Geometry: final body of the model. Coordinates: model frame, mm. Give positions to 0.01 mm unless a question says otherwise; leave off trailing zeros. Loops run counter-clockwise (first coordinate to the right, second up) from the corner with the lowest first, then second, coordinate; pieces in that order, holes last. Notation, with made-up numbers: (40.25, 24) -> (68.25, 24) arc R17 ccw to (68.25, 42) -> close; hole circle Ø4 at (38.25, 8.5). An arc over 180 degrees is marked (long way). One line per question, with ' | ' between items. Start each with the question number.
Item 1: Material intervals for line 1 along Z through (x, y) = (-26, 0.9); line 2 along X through (y, z) = (1.6, 88); line 3 along Z through (x, y) = (14, 1), sorted ascending. Write a range as [from, to].
Item 2: Section D-D on z = -68. Return loops of the section in (x, y).
Item 3: Section A-A on x = -85. Return loops of the section in (y, z).
Item 4: Section B-B on y = 0.55. Give the number of separate pieces and of enclosed holes in the cut face, then the cut area to 3 significant figures.
Item 5: Pin query (flat end, axial travel): P1, Ø5.5, axis at x = -14, z = -78, coming from the -Y side; P2, Ø1.5, axis at x = -86, y = 2.5, coming from the -Z side; P3, Ø3.5, axis at x = -103, z = -89, coming from the -Y side (1 decimal); P4, Ø1.5, axis at y = 1, z = 15.5, coming from the +X side. Return the tip coordinate at first contact, or that it passes through.
Item 6: Section C-C on z = 47. Return loops of the section in (x, y).
from build123d import *

# Parameters (mm, degrees)
SKETCH_1_R          = 2.1
EXTRUDE_1_DEPTH     = 3
FILLET_1_R          = 4
SKETCH_2_R          = 2.1
CUT_EXTRUDE_1_DEPTH = 4
EXTRUDE_2_DEPTH     = 3
FILLET_2_R          = 4
SKETCH_5_R          = 1.6
CUT_EXTRUDE_2_DEPTH = 4
FILLET_3_R          = 10
SKETCH_7_R          = 2.1
CUT_EXTRUDE_3_DEPTH = 4
CUT_EXTRUDE_4_DEPTH = 4


with BuildPart() as part:
    # 草图1 → 凸台-拉伸1 (new body)
    with BuildSketch(Plane(origin=(0, 0, 0), x_dir=(1, 0, 0), z_dir=(0, 1, 0))):
        with BuildLine():
            Line((-26, 93), (-96, 93))
            ThreePointArc((-96, 93), (-103.071067812, 95.928932188), (-106, 103))
            Line((-106, 103), (-106, 122.5))
            Line((-106, 122.5), (-130, 122.5))
            Line((-130, 122.5), (-130, -122.5))
            Line((-130, -122.5), (-106, -122.5))
            Line((-106, -122.5), (-106, -103))
            ThreePointArc((-106, -103), (-103.071067812, -95.928932188), (-96, -93))
            Line((-96, -93), (-26, -93))
            Line((-26, -93), (26, -93))
            Line((26, -93), (26, -73))
            Line((26, -73), (-76, -73))
            ThreePointArc((-76, -73), (-97.213203436, -64.213203436), (-106, -43))
            Line((-106, -43), (-106, 43))
            ThreePointArc((-106, 43), (-97.213203436, 64.213203436), (-76, 73))
            Line((-76, 73), (26, 73))
            Line((26, 73), (26, 93))
            Line((26, 93), (-26, 93))
        make_face()
        with Locations((-14, 88)):
            Circle(SKETCH_1_R, mode=Mode.SUBTRACT)
        with Locations((-14, 78)):
            Circle(SKETCH_1_R, mode=Mode.SUBTRACT)
        with Locations((14, 78)):
            Circle(SKETCH_1_R, mode=Mode.SUBTRACT)
        with Locations((14, 88)):
            Circle(SKETCH_1_R, mode=Mode.SUBTRACT)
        with Locations((14, -78)):
            Circle(SKETCH_1_R, mode=Mode.SUBTRACT)
        with Locations((14, -88)):
            Circle(SKETCH_1_R, mode=Mode.SUBTRACT)
        with Locations((-14, -78)):
            Circle(SKETCH_1_R, mode=Mode.SUBTRACT)
        with Locations((-14, -88)):
            Circle(SKETCH_1_R, mode=Mode.SUBTRACT)
    extrude(amount=EXTRUDE_1_DEPTH)

    # 圆角1
    fillet_1_edges = [part.edges().sort_by_distance(p)[0] for p in [
        (26, 1.5, -73),
        (26, 1.5, 73),
        (-130, 1.5, 122.5),
        (-130, 1.5, -122.5),
    ]]
    fillet(fillet_1_edges, radius=FILLET_1_R)

    # 草图2 → 切除-拉伸1 (cut, through all)
    with BuildSketch(Plane(origin=(0, 3, 0), x_dir=(1, 0, 0), z_dir=(0, 1, 0))):
        with Locations((-122, 118.5)):
            Circle(SKETCH_2_R)
        with Locations((-110, 118.5)):
            Circle(SKETCH_2_R)
        with Locations((-122, -118.5)):
            Circle(SKETCH_2_R)
        with Locations((-110, -118.5)):
            Circle(SKETCH_2_R)
    extrude(amount=-CUT_EXTRUDE_1_DEPTH, mode=Mode.SUBTRACT)

    # 草图4 → 凸台-拉伸2 (add)
    with BuildSketch(Plane(origin=(0, 3, 0), x_dir=(1, 0, 0), z_dir=(0, 1, 0))):
        Polygon((-106, 122.5), (16, 93), (-106, 93), align=None)
        Polygon((16, -93), (-106, -93), (-106, -122.5), align=None)
    extrude(amount=-EXTRUDE_2_DEPTH)

    # 圆角2
    fillet_2_edges = [part.edges().sort_by_distance(p)[0] for p in [
        (26, 1.5, 93),
        (-106, 1.5, 122.5),
        (-106, 1.5, -122.5),
        (26, 1.5, -93),
    ]]
    fillet(fillet_2_edges, radius=FILLET_2_R)

    # 草图5 → 切除-拉伸2 (cut, through all)
    with BuildSketch(Plane.XZ):
        with Locations((-110, -15)):
            Circle(SKETCH_5_R)
        with Locations((-110, -5)):
            Circle(SKETCH_5_R)
        with Locations((-110, 5)):
            Circle(SKETCH_5_R)
        with Locations((-110, 15)):
            Circle(SKETCH_5_R)
        with Locations((-26, -77)):
            Circle(SKETCH_5_R)
        with Locations((-36, -77)):
            Circle(SKETCH_5_R)
        with Locations((-46, -77)):
            Circle(SKETCH_5_R)
        with Locations((-56, -77)):
            Circle(SKETCH_5_R)
        with Locations((-56, 77)):
            Circle(SKETCH_5_R)
        with Locations((-46, 77)):
            Circle(SKETCH_5_R)
        with Locations((-36, 77)):
            Circle(SKETCH_5_R)
        with Locations((-26, 77)):
            Circle(SKETCH_5_R)
    extrude(amount=-CUT_EXTRUDE_2_DEPTH, mode=Mode.SUBTRACT)

    # 圆角3
    fillet_3_edges = [part.edges().sort_by_distance(p)[0] for p in [
        (16, 1.5, -93),
        (16, 1.5, 93),
    ]]
    fillet(fillet_3_edges, radius=FILLET_3_R)

    # 草图7 → 切除-拉伸3 (cut, through all)
    with BuildSketch(Plane(origin=(0, 3, 0), x_dir=(1, 0, 0), z_dir=(0, 1, 0))):
        with Locations((-123, -74)):
            Circle(SKETCH_7_R)
        with Locations((-103, -74)):
            Circle(SKETCH_7_R)
        with Locations((-103, -89)):
            Circle(SKETCH_7_R)
        with Locations((-123, -89)):
            Circle(SKETCH_7_R)
        with Locations((-123, 89)):
            Circle(SKETCH_7_R)
        with Locations((-103, 89)):
            Circle(SKETCH_7_R)
        with Locations((-103, 74)):
            Circle(SKETCH_7_R)
        with Locations((-123, 74)):
            Circle(SKETCH_7_R)
    extrude(amount=-CUT_EXTRUDE_3_DEPTH, mode=Mode.SUBTRACT)

    # 草图8 → 切除-拉伸4 (cut, through all)
    with BuildSketch(Plane(origin=(0, 3, 0), x_dir=(1, 0, 0), z_dir=(0, 1, 0))):
        with BuildLine():
            Line((-99.173057144, 103.191305263), (-95.290856101, 86.83060087))
            ThreePointArc((-95.290856101, 86.83060087), (-93.457663057, 84.008976045), (-90.251444241, 82.988033197))
            Line((-90.251444241, 82.988033197), (-38.266720564, 84.80337975))
            ThreePointArc((-38.266720564, 84.80337975), (-33.471381612, 89.251949162), (-37.181429777, 94.639025187))
            Line((-37.181429777, 94.639025187), (-93.048354496, 109.184383027))
            ThreePointArc((-93.048354496, 109.184383027), (-97.805066963, 107.919418235), (-99.173057144, 103.191305263))
        make_face()
        with BuildLine():
            Line((-109, 86.75), (-117, 86.75))
            ThreePointArc((-117, 86.75), (-119.121320344, 85.871320344), (-120, 83.75))
            Line((-120, 83.75), (-120, 79.25))
            ThreePointArc((-120, 79.25), (-119.121320344, 77.128679656), (-117, 76.25))
            Line((-117, 76.25), (-109, 76.25))
            ThreePointArc((-109, 76.25), (-106.878679656, 77.128679656), (-106, 79.25))
            Line((-106, 79.25), (-106, 83.75))
            ThreePointArc((-106, 83.75), (-106.878679656, 85.871320344), (-109, 86.75))
        make_face()
        with BuildLine():
            Line((-109, -76.25), (-117, -76.25))
            ThreePointArc((-117, -76.25), (-119.121320344, -77.128679656), (-120, -79.25))
            Line((-120, -79.25), (-120, -83.75))
            ThreePointArc((-120, -83.75), (-119.121320344, -85.871320344), (-117, -86.75))
            Line((-117, -86.75), (-109, -86.75))
            ThreePointArc((-109, -86.75), (-106.878679656, -85.871320344), (-106, -83.75))
            Line((-106, -83.75), (-106, -79.25))
            ThreePointArc((-106, -79.25), (-106.878679656, -77.128679656), (-109, -76.25))
        make_face()
        with BuildLine():
            Line((-115.138114684, 115), (-115.716605496, 115))
            ThreePointArc((-115.716605496, 115), (-117.80168228, 114.156954985), (-118.714883338, 112.101636537))
            Line((-118.714883338, 112.101636537), (-119.274205372, 95.601636537))
            ThreePointArc((-119.274205372, 95.601636537), (-118.432882515, 93.414923216), (-116.27592753, 92.5))
            Line((-116.27592753, 92.5), (-111.222860446, 92.5))
            ThreePointArc((-111.222860446, 92.5), (-108.869363513, 93.639609669), (-108.30391182, 96.192631877))
            Line((-108.30391182, 96.192631877), (-112.219166057, 112.692631877))
            ThreePointArc((-112.219166057, 112.692631877), (-113.277724353, 114.353496934), (-115.138114684, 115))
        make_face()
        with BuildLine():
            Line((-37.181429777, -94.639025187), (-93.048354496, -109.184383027))
            ThreePointArc((-93.048354496, -109.184383027), (-97.805066963, -107.919418235), (-99.173057144, -103.191305263))
            Line((-99.173057144, -103.191305263), (-95.290856101, -86.83060087))
            ThreePointArc((-95.290856101, -86.83060087), (-93.457663057, -84.008976045), (-90.251444241, -82.988033197))
            Line((-90.251444241, -82.988033197), (-38.266720564, -84.80337975))
            ThreePointArc((-38.266720564, -84.80337975), (-33.471381612, -89.251949162), (-37.181429777, -94.639025187))
        make_face()
        with BuildLine():
            Line((-112.219166057, -112.692631877), (-108.30391182, -96.192631877))
            ThreePointArc((-108.30391182, -96.192631877), (-108.869363513, -93.639609669), (-111.222860446, -92.5))
            Line((-111.222860446, -92.5), (-116.27592753, -92.5))
            ThreePointArc((-116.27592753, -92.5), (-118.432882515, -93.414923216), (-119.274205372, -95.601636537))
            Line((-119.274205372, -95.601636537), (-118.714883338, -112.101636537))
            ThreePointArc((-118.714883338, -112.101636537), (-117.80168228, -114.156954985), (-115.716605496, -115))
            Line((-115.716605496, -115), (-115.138114684, -115))
            ThreePointArc((-115.138114684, -115), (-113.277724353, -114.353496934), (-112.219166057, -112.692631877))
        make_face()
    extrude(amount=-CUT_EXTRUDE_4_DEPTH, mode=Mode.SUBTRACT)


solid = part.part
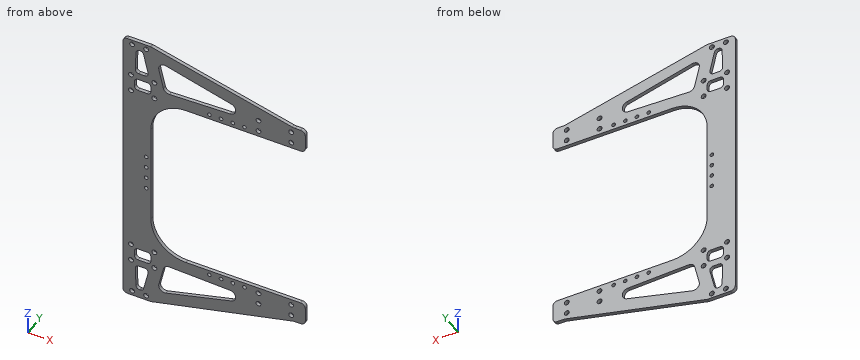
Result sheet:
1) line 1: z = [-103.16, -78.6], [-75.4, -73], [73, 75.4], [78.6, 103.16] | line 2: x = [-130, -124.85], [-121.15, -104.85], [-101.15, -95.57], [-33.78, -16.1], [-11.9, 11.9], [16.1, 26] | line 3: z = [-93.48, -90.1], [-85.9, -80.1], [-75.9, -73], [73, 75.9], [80.1, 85.9], [90.1, 93.48]
2) outline: (-130, 0) -> (-92.58, 0) -> (-92.58, 3) -> (-130, 3) -> close
3) outline: (0, -117.42) -> (3, -117.42) -> (3, -107.09) -> (0, -107.09) -> close; (0, -83.17) -> (3, -83.17) -> (3, -71.62) -> (0, -71.62) -> close; (0, 71.62) -> (3, 71.62) -> (3, 83.17) -> (0, 83.17) -> close; (0, 107.09) -> (3, 107.09) -> (3, 117.42) -> (0, 117.42) -> close
4) separate pieces: 1 | enclosed holes: 38 | area: 11,800 mm²
5) P1: stops at y = 0 | P2: stops at z = -117.85 | P3: passes through | P4: stops at x = -106
6) outline: (-130, 0) -> (-105.73, 0) -> (-105.73, 3) -> (-130, 3) -> close
